For this review, take the finished solid that the model builds, in its own axes (mm). Face numbers are marked on the shaded views. A direction names the side the tool comes from. Give positions to 0.01 mm unless a question says otherwise; leave off trailing zeros. Loops run counter-clockwise (first coordinate to the right, second up) from the corner with the lowest first, then second, coordinate; pieces in that order, holes last. Notation, with made-up numbers: (-34.5, 26) - (20.5, 26) arc R32 ccw to (20.5, 54) - close; hole circle Ø1 at (30.5, 77.5). An arc over 180 degrees is marked (long way). Use CSV: the item, a comma, the result in double quotes. Start each with the question number.
1. Take a section at A-A on z = 3.25. Give the boundary of the cut face in (x, y), plus the area to 3 significant figures.
2. Take a section at D-D on y = 4. Give the boundary of the cut face in (x, z), plus the area to 3 significant figures.
3. Mouldability with a two-part tool opening along X and no side actions: class the marked faces 3, 4, 5 and 6 as pulls with the +X half, pulls with the -X half, needs draft (parallel to the pull), parting line crosses it, or undercut.
4. For pin 1 (1.4 mm diameter, centred on x = -1, y = -0.5, fed in from +Z), flat-tipped, find the tip position at first contact; note if it passes through.
5. Take a section at C-C on x = 4. Give the boundary of the cut face in (y, z), plus the area to 3 significant figures.
6. Take a section at B-B on y = 0. Give the boundary of the cut face in (x, z), plus the area to 3 significant figures.
7. For the marked faces 1 and 2, list the 3-axis set-ups (+Z, -Z, +X, -X, +Y, -Y) from which the entire face can be reached by the end or side of a thin tool; tool diameter is ignored.
8. Wall thickness on line 1 (X direction, y = -8, z = 3.5); line 2 (Y direction, x = 4.25, z = 8.75); line 3 (X direction, y = 12, z = 8): over which ranges is each line inside the solid? List them lowest first.
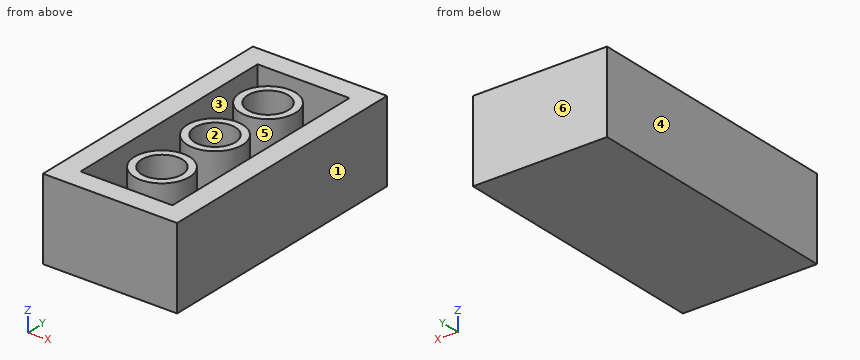
```python
from build123d import *

# Parameters (mm, degrees)
F0_W     = 15.8877
F0_H     = 9.5504
F1_DEPTH = 7.9121
F4_T     = -2.4892
F5_R     = 3.2512
F5_R_2   = 2.4003
F6_DEPTH = 7.0612


with BuildPart() as f1:
    # F0 (on Right) → F1 (new body)
    with BuildSketch(Plane.YZ):
        with Locations((7.94385, 4.7752)):
            Rectangle(F0_W, F0_H)
    extrude(amount=F1_DEPTH)

    # F2: F1 across plane


with BuildPart() as f1_1:
    add(f1.part)
    add(f1.part.mirror(Plane.XZ))

    # F3: F1 across plane


with BuildPart() as f1_2:
    add(f1_1.part)
    add(f1_1.part.mirror(Plane.YZ))

    # F4
    f4_openings = [f1_2.faces().sort_by_distance(p)[0] for p in [
        (0, 0, 9.5504),
    ]]
    offset(amount=F4_T, openings=f4_openings)

    # F5 (on face) → F6 (join, through all)
    with BuildSketch(Plane.XY.offset(2.4892)):
        with Locations((0, -8.0264)):
            Circle(F5_R)
        with Locations((0, -8.0264)):
            Circle(F5_R_2, mode=Mode.SUBTRACT)
        Circle(F5_R)
        Circle(F5_R_2, mode=Mode.SUBTRACT)
        with Locations((0, 8.0264)):
            Circle(F5_R)
        with Locations((0, 8.0264)):
            Circle(F5_R_2, mode=Mode.SUBTRACT)
    extrude(amount=F6_DEPTH)


solid = f1_2.part
```
Check result:
1,outline,"(-7.91, -15.89) - (7.91, -15.89) - (7.91, 15.89) - (-7.91, 15.89) - close; circle Ø6.5 at (0, -8.03); circle Ø6.5 at (0, 0); circle Ø6.5 at (0, 8.03); hole (-5.42, -13.4) - (5.42, -13.4) - (5.42, 13.4) - (-5.42, 13.4) - close; hole circle Ø4.8 at (0, -8.03); hole circle Ø4.8 at (0, 0); hole circle Ø4.8 at (0, 8.03)"
1,area,"258 mm²"
2,outline,"(-7.91, 0) - (7.91, 0) - (7.91, 9.55) - (5.42, 9.55) - (5.42, 2.49) - (-5.42, 2.49) - (-5.42, 9.55) - (-7.91, 9.55) - close"
2,area,"74.5 mm²"
3,face 3,"undercut"
3,face 4,"pulls with the -X half"
3,face 5,"undercut"
3,face 6,"needs draft"
4,pin 1,"stops at z = 2.49"
5,outline,"(-15.89, 0) - (15.89, 0) - (15.89, 9.55) - (13.4, 9.55) - (13.4, 2.49) - (-13.4, 2.49) - (-13.4, 9.55) - (-15.89, 9.55) - close"
5,area,"114 mm²"
6,outline,"(-7.91, 0) - (7.91, 0) - (7.91, 9.55) - (5.42, 9.55) - (5.42, 2.49) - (3.25, 2.49) - (3.25, 9.55) - (2.4, 9.55) - (2.4, 2.49) - (-2.4, 2.49) - (-2.4, 9.55) - (-3.25, 9.55) - (-3.25, 2.49) - (-5.42, 2.49) - (-5.42, 9.55) - (-7.91, 9.55) - close"
6,area,"86.6 mm²"
7,face 1,"+Z, -Z, +X, +Y, -Y"
7,face 2,"+Z"
8,line 1,"x = -7.91 to -5.42, -3.25 to -2.4, 2.4 to 3.25, 5.42 to 7.91"
8,line 2,"y = -15.89 to -13.4, 13.4 to 15.89"
8,line 3,"x = -7.91 to -5.42, 5.42 to 7.91"
